Geometry: final body of the model. Coordinates: model frame, mm. Face numbers are marked on the shaded views. A direction names the side the tool comes from. Round coordinates to 2 decimals unless told otherwise and drop trailing zeros. Write each loop counter-clockwise with the first axis right and the second up, starting at its lowest first coordinate (ties: lowest second). Pieces come first, ordered by that corner, then holes. Notation, with made-up numbers: M -30,-31 L -16,-31 A22 ccw -16,-1 Z; hole C 11,0.5 d7. An arc over 180 degrees is marked long. Answer as CSV lines item,"result". Start each with the question number.
Q1. Ray query, probe 1 along Y at (x, z) = (10, 1.8); probe 2 along Y at (x, z) = (-7.5, 23.5); probe 3 along X at (y, z) = (-1, 7.5). Return the intervals inside material, ascending.
Q2. Section query C-C on z = 5.5. Output: boundary loops of the cut face in (x, y).
Q3. First-contact query: pin 1 (12.5 mm diameter, centred on x = 0.5, z = 16, fed in from +Y); pin 2 (7 mm diameter, centred on x = 0.5, z = 15.5, fed in from -Y); pin 3 (2 mm diameter, centred on x = 10.5, z = 19, fed in from +Y); pin 4 (3 mm diameter, centred on x = 10, y = -10, fed in from +Z). Flat tips, straight axial feed; report the tip coordinate or a pass-through.
Q4. Section query A-A on y = -19. Output: boundary loops of the cut face in (x, z), and give its area (3 significant figures).
Q5. Section query B-B on x = 10. Output: boundary loops of the cut face in (y, z).
Q6. Reachability of the marked faces 1, 2, 3, 4 and 5 from +Z, -Z, +X, -X, +Y, -Y: full face, straight path, thin tool, end or side. Return the list, or none.
Q7. Section query D-D on y = 10. Output: boundary loops of the cut face in (x, z), and give its area (3 significant figures).
```python
from build123d import *

# Parameters (mm, degrees)
SKETCH1_W                       = 30
SKETCH1_H                       = 32
BOSS_EXTRUDE1_DEPTH             = 5
M3_CLEARANCE_HOLE1_D            = 3.4
SKETCH5_W                       = 25.4
SKETCH5_H                       = 30.4
BOSS_EXTRUDE2_DEPTH             = 5
BOSS_EXTRUDE3_REACH             = 38.377
SKETCH8_W                       = 5
SKETCH8_H                       = 10
BOSS_EXTRUDE3_DIRECTION_2_REACH = 38.377
SKETCH10_W                      = 6.4
SKETCH10_H                      = 19.2
CUT_EXTRUDE1_DEPTH              = 2.7
FILLET1_R                       = 1
SKETCH12_W                      = 25.4
SKETCH12_H                      = 4.8
BOSS_EXTRUDE5_DEPTH             = 5
FILLET2_START                   = -1
FILLET2_DEPTH                   = 30.4
FILLET2_2_DEPTH                 = 5


with BuildPart() as part:
    # Sketch1 → Boss-Extrude1 (new body)
    with BuildSketch(Plane.XY):
        Rectangle(SKETCH1_W, SKETCH1_H)
    extrude(amount=BOSS_EXTRUDE1_DEPTH)

    # M3 Clearance Hole1 (through all)
    with Locations(Plane.XY.offset(5)):
        with Locations((-10, 10), (10, 10), (10, -10), (-10, -10)):
            Hole(M3_CLEARANCE_HOLE1_D / 2)

    # Sketch5 → Boss-Extrude2 (add)
    with BuildSketch(Plane.XZ.offset(16)):
        with Locations((0, 15.2)):
            Rectangle(SKETCH5_W, SKETCH5_H)
    extrude(amount=BOSS_EXTRUDE2_DEPTH)

    # Boss-Extrude3: up to this plane
    boss_extrude3_end = Plane(origin=(0, -16, 0), z_dir=(0, -1, 0))
    # Sketch8 → Boss-Extrude3 (add, up to the surface)
    with BuildSketch(Plane(origin=(0, -10.5, 10.5), x_dir=(1, 0, 0), z_dir=(0, -0.7071067811865475, 0.7071067811865477)), mode=Mode.PRIVATE) as boss_extrude3_sk1:
        Rectangle(SKETCH8_W, SKETCH8_H)
    boss_extrude3_tool1 = split(extrude(boss_extrude3_sk1.sketch, amount=BOSS_EXTRUDE3_REACH, mode=Mode.PRIVATE), bisect_by=boss_extrude3_end, keep=Keep.BOTH, mode=Mode.PRIVATE)
    add(boss_extrude3_tool1.solids().sort_by_distance((0, -10.5, 10.5))[0])

    # Boss-Extrude3 direction 2: up to this plane
    boss_extrude3_direction_2_end = Plane(origin=(0, 0, 5), z_dir=(0, 0, 1))
    # Sketch8 → Boss-Extrude3 direction 2 (add, up to the surface)
    with BuildSketch(Plane(origin=(0, -10.5, 10.5), x_dir=(1, 0, 0), z_dir=(0, -0.7071067811865475, 0.7071067811865477)), mode=Mode.PRIVATE) as boss_extrude3_direction_2_sk1:
        Rectangle(SKETCH8_W, SKETCH8_H)
    boss_extrude3_direction_2_tool1 = split(extrude(boss_extrude3_direction_2_sk1.sketch, amount=-BOSS_EXTRUDE3_DIRECTION_2_REACH, mode=Mode.PRIVATE), bisect_by=boss_extrude3_direction_2_end, keep=Keep.BOTH, mode=Mode.PRIVATE)
    add(boss_extrude3_direction_2_tool1.solids().sort_by_distance((0, -10.5, 10.5))[0])

    # Sketch10 → Cut-Extrude1 (cut)
    with BuildSketch(Plane.XZ.offset(21)):
        with Locations((0, 14.6)):
            Rectangle(SKETCH10_W, SKETCH10_H)
    extrude(amount=-CUT_EXTRUDE1_DEPTH, mode=Mode.SUBTRACT)

    # Fillet1
    fillet1_edges = [part.edges().sort_by_distance(p)[0] for p in [
        (12.7, -18.5, 30.4),
        (-12.7, -18.5, 30.4),
    ]]
    fillet(fillet1_edges, radius=FILLET1_R)

    # Sketch12 → Boss-Extrude5 (add)
    with BuildSketch(Plane.XZ.offset(21)):
        with Locations((0, 2.4)):
            Rectangle(SKETCH12_W, SKETCH12_H)
    extrude(amount=BOSS_EXTRUDE5_DEPTH)

    # Fillet2: read off the stored shape, not the designer's step
    # Fillet2 outline → Fillet2 (cut)
    with BuildSketch(Plane.XY.offset(FILLET2_START)):
        with BuildLine():
            Line((15, -16), (15, -14.9))
            ThreePointArc((15, -14.9), (14.677817459, -15.677817459), (13.9, -16))
            Line((13.9, -16), (15, -16))
        make_face()
        with BuildLine():
            Line((-15, -16), (-13.9, -16))
            ThreePointArc((-13.9, -16), (-14.677817459, -15.677817459), (-15, -14.9))
            Line((-15, -14.9), (-15, -16))
        make_face()
    extrude(amount=FILLET2_DEPTH, mode=Mode.SUBTRACT)

    # Fillet2 2 outline → Fillet2 2 (add)
    with BuildSketch(Plane.XY):
        with BuildLine():
            ThreePointArc((12.7, -17.1), (13.022182541, -16.322182541), (13.8, -16))
            Line((13.8, -16), (12.7, -16))
            Line((12.7, -16), (12.7, -17.1))
        make_face()
        with BuildLine():
            Line((-12.7, -16), (-13.8, -16))
            ThreePointArc((-13.8, -16), (-13.022182541, -16.322182541), (-12.7, -17.1))
            Line((-12.7, -17.1), (-12.7, -16))
        make_face()
    extrude(amount=FILLET2_2_DEPTH)


solid = part.part
```
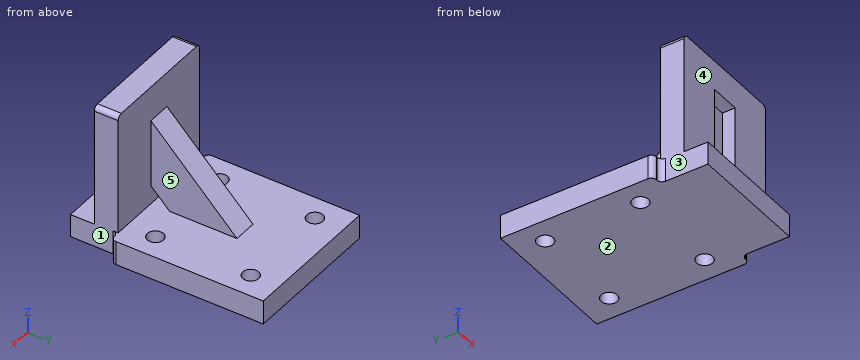
Entries:
1,probe 1,"y = -26 to -11.7, -8.3 to 8.3, 11.7 to 16"
1,probe 2,"y = -21 to -16"
1,probe 3,"x = -2.5 to 2.5"
2,outline,"M -12.7,-21 L -3.2,-21 L -3.2,-18.3 L 3.2,-18.3 L 3.2,-21 L 12.7,-21 L 12.7,-16 L -12.7,-16 Z; M -2.5,-12.57 L 2.5,-12.57 L 2.5,1.57 L -2.5,1.57 Z"
3,pin 1,"stops at y = -2.68"
3,pin 2,"stops at y = -21"
3,pin 3,"stops at y = -16"
3,pin 4,"passes through"
4,outline,"M -12.7,0 L 12.7,0 L 12.7,29.4 A1 ccw 11.7,30.4 L -11.7,30.4 A1 ccw -12.7,29.4 Z; hole M -3.2,5 L 3.2,5 L 3.2,24.2 L -3.2,24.2 Z"
4,area,"649 mm^2"
5,outline,"M -26,0 L -11.7,0 L -11.7,5 L -16,5 L -16,30.4 L -21,30.4 L -21,4.8 L -26,4.8 Z; M -8.3,0 L 8.3,0 L 8.3,5 L -8.3,5 Z; M 11.7,0 L 16,0 L 16,5 L 11.7,5 Z"
6,face 1,"+Z, +X, -Y"
6,face 2,"-Z, +X, -X, +Y, -Y"
6,face 3,"+Z, -X, -Y"
6,face 4,"+Z, +X, -X, -Y"
6,face 5,"+Z, +X, +Y"
7,outline,"M -15,0 L -11.7,0 L -11.7,5 L -15,5 Z; M -8.3,0 L 8.3,0 L 8.3,5 L -8.3,5 Z; M 11.7,0 L 15,0 L 15,5 L 11.7,5 Z"
7,area,"116 mm^2"
